Geometry check sheet. Reference: the model listing, model coordinates, mm. Face numbers are marked on the shaded views. A direction names the side the tool comes from. Give positions to 0.01 mm unless a question says otherwise; leave off trailing zeros. Order: outer loops, then holes, each group sorted by start corner. A loop starts at its lowest first (then second) coordinate and runs counter-clockwise, first axis right, second up. Notation, with made-up numbers: M -33,-39 L -28,-39 A22 ccw -28,-23 Z; hole C 79.25,56 d6. An arc over 180 degrees is marked long. Put each result on its own line as item: value. Start each with the question number.
Q1. Section check C-C on z = 11.5. Record the cut outline in (x, y).
Q2. Material ranges on L1, parallel to X at y = 0.5, z = 8.25; L2, parallel to Z at x = 23, y = 18 (3 decimals); L3, parallel to Y at x = -5.5, z = 10.5, recorded low to high.
Q3. Section check A-A on y = 0. Record the cut outline in (x, z) (3 decimals).
Q4. Section check B-B on z = 1.5. Record the cut outline in (x, y) (3 decimals), then the cut area to 3 significant figures.
Q5. Access from +Z, -Z, +X, -X, +Y, -Y to the whole of each face (thin tool, end or side, straight path). Record for the marked faces 1 and 2.
Q6. Section check D-D on x = 20.5. Record the cut outline in (y, z) (3 decimals), then the cut area to 3 significant figures.
Q7. Go/stop test with flat-tipped pins: pin 1 (8 mm diameter, centred on x = -1.5, z = 10.5, fed in from +Y); pin 2 (5 mm diameter, centred on x = -28.01, y = 20.86, fed in from +Z); pin 3 (10 mm diameter, centred on x = -7.5, y = 24, fed in from +Z) (3 decimals); pin 4 (2 mm diameter, centred on y = 2, z = 16, fed in from +X). Record where each tip stops, or that it passes through.
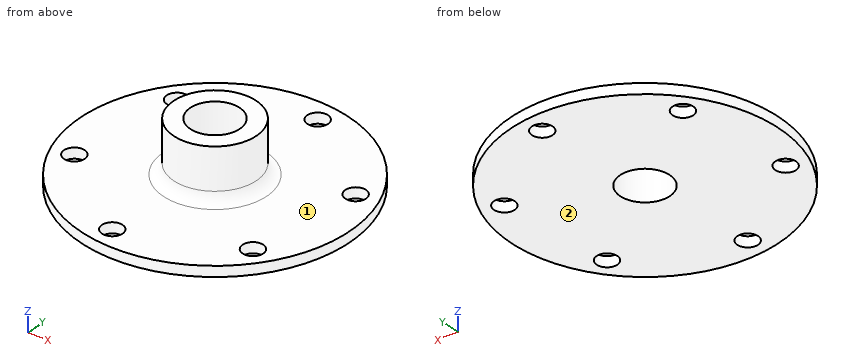
```python
from build123d import *

# Parameters (mm, degrees)
SKETCH3_R          = 7.62
SKETCH3_R_2        = 3.175
CUT_EXTRUDE1_DEPTH = 62.401577748
CIRPATTERN1_COUNT  = 6
FILLET1_R          = 3.175


with BuildPart() as part:
    # Sketch2 → Revolve1 (revolve)
    with BuildSketch(Plane(origin=(0, 0, 0), x_dir=(0, 0, -1), z_dir=(1, 0, 0))):
        Polygon((0, 0), (0, 41.275), (-3.175, 41.275), (-3.175, 12.7), (-19.05, 12.7), (-19.05, 0), align=None)
    revolve(axis=Axis((0, 0, 0), (0, 0, 1)))

    # Sketch3 → Cut-Extrude1 (cut, through all)
    with BuildSketch(Plane.XY.offset(19.05)):
        Circle(SKETCH3_R)
        with Locations((-28.008609796, 20.863206903)):
            Circle(SKETCH3_R_2)
    cut_extrude1 = extrude(amount=-CUT_EXTRUDE1_DEPTH, mode=Mode.SUBTRACT)

    # CirPattern1: Cut-Extrude1 ×6 about axis
    cirpattern1_axis = Axis((0, 0, 0), (0, 0, 1))
    for i in range(1, CIRPATTERN1_COUNT):
        add(cut_extrude1.rotate(cirpattern1_axis, i * 360 / CIRPATTERN1_COUNT), mode=Mode.SUBTRACT)

    # Fillet1
    fillet1_edges = [part.edges().sort_by_distance(p)[0] for p in [
        (0, -12.7, 3.175),
    ]]
    fillet(fillet1_edges, radius=FILLET1_R)


solid = part.part
```
Results found:
1. outline: C 0,0 d25.4; hole C 0,0 d15.24
2. L1: x = -12.69 to -7.6, 7.6 to 12.69
2. L2: z = 0 to 3.175
2. L3: y = -11.45 to -5.27, 5.27 to 11.45
3. outline: M -41.275,0 L -7.62,0 L -7.62,19.05 L -12.7,19.05 L -12.7,6.35 A3.175 cw -15.875,3.175 L -41.275,3.175 Z; M 7.62,0 L 41.275,0 L 41.275,3.175 L 15.875,3.175 A3.175 cw 12.7,6.35 L 12.7,19.05 L 7.62,19.05 Z
4. outline: C 0,0 d82.55; hole C -32.072,-13.825 d6.35; hole C -28.009,20.863 d6.35; hole C 0,0 d15.24; hole C -4.064,-34.688 d6.35; hole C 4.064,34.688 d6.35; hole C 28.009,-20.863 d6.35; hole C 32.072,13.825 d6.35
4. area: 4,980 mm^2
5. face 1: +Z
5. face 2: -Z, +X, -X, +Y, -Y
6. outline: M -35.824,0 L 35.824,0 L 35.824,3.175 L -35.824,3.175 Z
6. area: 227 mm^2
7. pin 1: stops at y = 12.7
7. pin 2: passes through
7. pin 3: stops at z = 3.175
7. pin 4: stops at x = 12.66
